Autodesk Inventor part; units mm, degrees
ref_plane "YZ Plane" through (0, 0, 0) normal (1, 0, 0) x (0, 1, 0)
ref_plane "XZ Plane" through (0, 0, 0) normal (0, 1, 0) x (-1, 0, 0)
ref_plane "XY Plane" through (0, 0, 0) normal (0, 0, 1) x (1, 0, 0)
sketch "Sketch1" plane through (0, 0, 0) normal (0, 0, 1) x (1, 0, 0)
  line L0 (0, 0) -> (75, 0)
  line L1 (75, 0) -> (75, -105)
  line L2 (75, -105) -> (0, -105)
  line L3 (0, -105) -> (0, 0)
  dimension "d0" = 75
  dimension "d1" = 105
extrude "Extrusion1" add sketch "Sketch1" along normal blind 5
sketch "Sketch2" plane through (75, -105, 0) normal (1, 0, 0) x (0, 0, -1)
  line L0 (-5, 0) -> (-5, 105)
  line L1 (0, 0) -> (0, 105)
  line L2 (-5, 105) -> (0, 105)
  line L3 (0, 105) -> (0, 102)
  line L4 (0, 102) -> (-5, 102)
  line L5 (-5, 102) -> (-5, 105)
  circle A0 centre (-2.5, 103) radius 1.75
  line L6 (0, 105) -> (-1, 105)
  line L7 (0, 105) -> (-5, 105)
  line L8 (0, 105) -> (0, 104)
  line L9 (-1, 105) -> (0, 104)
  point P0 (-1, 105)
  point P1 (0, 104)
  point P2 (-2.5, 105)
  point P3 (-2.5, 105)
  dimension "d4" = 3
  dimension "d5" = 3.5
  dimension "d6" = 1
  dimension "d7" = 1
  dimension "d14" = 2
extrude "Extrusion2" cut sketch "Sketch2" against normal through all contours A0 L4 | L4 A0
extrude "Extrusion3" cut sketch "Sketch2" against normal through all contours L2 L1 L9
sketch "Sketch3" plane through (75, -105, 5) normal (1, 0, 0) x (0, 0, -1)
  line L0 (0, 105) -> (0, 0)
  line L1 (5, 104) -> (5, 0)
  line L2 (0, 0) -> (5, 2.3157)
  line L3 (5, 0) -> (5, 104)
  line L4 (5, 0) -> (0, 0)
  line L5 (5, 2.3157) -> (5, 0)
  line L6 (5, 0) -> (0, 0)
  point P0 (5, 105)
extrude "Extrusion4" cut sketch "Sketch3" against normal through all
properties part number "stojka - správná verze"
Can you work these out from the model? Positions are in its coordinate system, mm. Round coordinates to 2 decimals unless told otherwise and drop trailing zeros. Loops run counter-clockwise (first coordinate to the right, second up) from the corner with the lowest first, then second, coordinate; pieces in that order, holes last. Notation, with made-up numbers: M 18.25,-9.5 L 65.25,-9.5 A5 ccw 65.25,-1.5 Z; hole C 79,-30 d3. An arc over 180 degrees is marked long. Write item = value, one per line. Start each with the question number.
(1) Suppose I cut it at A-A on z = 2.5. Write out the boundary of the cut face in (x, y).
(2) Suppose I cut it at B-B on x = 9. Write out the boundary of the cut face in (y, z).
(3) I'm going to push flat-ended pins straight in: P1, Ø1, axis at x = 35, z = 2.5, coming from the +Y side; P2, Ø2, axis at y = -2, z = 2.5, coming from the +X side. Where does each tip first touch, or does it pass through?
(4) If we mould it in two halves opening along Y, with no side actions, what happens to faces 1 (the face through (37, 0, 3)), 2 (the face through (38.025, -2.67, 0.883)), 3 (the face through (0, -53, 2))? For each: released by +Y, released by -Y, zero draft, split by the parting line, or undercut.
(5) I need wall thicknesses on line 1 along Z through (x, y) = (37.5, -2); line 2 along Y through (x, z) = (49.5, 3.65); line 3 along Y through (x, z) = (16.5, 2.5). Which ranges of each line are inside material? Lowest first, please.
Answer block:
q1.outline = M 0,-103.84 L 75,-103.84 L 75,-3.75 L 0,-3.75 Z; M 0,-0.25 L 75,-0.25 L 75,0 L 0,0 Z
q2.outline = M -105,5 L -102.68,0 L -1,0 L 0,1 L 0,5 Z; hole C -2,2.5 d3.5
q3.P1 = 0
q3.P2 = through
q4.face_1 = released by +Y
q4.face_2 = undercut
q4.face_3 = zero draft
q5.line_1 = 0 to 0.75, 4.25 to 5
q5.line_2 = -104.37 to -3.32, -0.68 to 0
q5.line_3 = -103.84 to -3.75, -0.25 to 0
